from build123d import *

# Parameters (mm, degrees)
F0_W         = 70
F0_H         = 20
F0_R         = 5.25
F1_DEPTH     = 17.5
F2_T         = -3
F3_W         = 80
F3_H         = 53
F4_DEPTH     = 25
F5_T         = 2.5
F5_T3_DEPTH  = 40
F5_T5_DEPTH  = 75
F5_T7_DEPTH  = 69
F5_T9_DEPTH  = 22
F5_T11_DEPTH = 34


# Not quite as in the source:
# - a shell that OpenCascade refuses in one call is made with other operations: the cavity is built on its own and cut out


with BuildPart() as f1:
    # F0 (on Right) → F1 (new body, symmetric)
    with BuildSketch(Plane.YZ):
        Rectangle(F0_W, F0_H)
        with Locations((-22.5, 0)):
            Circle(F0_R, mode=Mode.SUBTRACT)
        with Locations((22.5, 0)):
            Circle(F0_R, mode=Mode.SUBTRACT)
    extrude(amount=F1_DEPTH, both=True)

    # F2
    f2_openings = [f1.faces().sort_by_distance(p)[0] for p in [
        (0, 0, 10),
        (0, -27.75, 0),
        (0, 17.25, 0),
    ]]
    offset(amount=F2_T, openings=f2_openings)

    # F3 (on Right) → F4 (join, symmetric)
    with BuildSketch(Plane.YZ):
        with Locations((0, 36.5)):
            Rectangle(F3_W, F3_H)
    extrude(amount=F4_DEPTH, both=True)

    # F5: shell of thickness 2.5, made by hand


with BuildPart() as f5_core1:
    # F5_t2: copy of F1
    add(f1.part)

    # the walls: a layer under each face that stays
    f5_faces = [f5_core1.faces().sort_by_distance(p)[0] for p in [
        (-21.4285714286, -34.2857142857, 10),
        (-25, 0, 36.5),
        (0, -40, 36.5),
        (0, 40, 36.5),
        (25, 0, 36.5),
        (0, 35, 0),
        (17.5, 0, 0),
        (0, -35, 0),
        (-17.5, 0, 0),
        (0, 0, -10),
        (16, -27.75, 0),
        (16, 17.25, 0),
        (-16, -27.75, 0),
        (-16, 17.25, 0),
        (14.5, 0, 1.5),
        (-14.5, 0, 1.5),
        (0, 0, 10),
        (0, -32, 1.5),
        (0, 0, -7),
        (0, 32, 1.5),
    ]]
    thicken(f5_faces, amount=-F5_T, mode=Mode.SUBTRACT)

    # F5_s4 → F5_t3 (cut)
    with BuildSketch(Plane.YZ.offset(-20)):
        Polygon((35.025, 9.975), (35, 12.5), (32.5, 12.5), (32.5, 10), align=None)
        Polygon((-35.025, 9.975), (-35, 12.5), (-32.5, 12.5), (-32.5, 10), align=None)
    extrude(amount=F5_T3_DEPTH, mode=Mode.SUBTRACT)

    # F5_s6 → F5_t5 (cut)
    with BuildSketch(Plane.XZ.offset(-37.5)):
        Polygon((17.525, 9.975), (17.5, 12.5), (15, 12.5), (15, 10), align=None)
        Polygon((-17.525, 9.975), (-17.5, 12.5), (-15, 12.5), (-15, 10), align=None)
    extrude(amount=F5_T5_DEPTH, mode=Mode.SUBTRACT)

    # F5_s8 → F5_t7 (cut)
    with BuildSketch(Plane.XZ.offset(-34.5)):
        Polygon((14.475, 9.975), (17, 10), (17, 12.5), (14.5, 12.5), align=None)
        Polygon((14.475, -6.975), (17, -7), (17, -9.5), (14.5, -9.5), align=None)
        Polygon((-14.475, 9.975), (-17, 10), (-17, 12.5), (-14.5, 12.5), align=None)
        Polygon((-14.475, -6.975), (-17, -7), (-17, -9.5), (-14.5, -9.5), align=None)
    extrude(amount=F5_T7_DEPTH, mode=Mode.SUBTRACT)

    # F5_s10 → F5_t9 (cut)
    with BuildSketch(Plane.XY.offset(-9.5)):
        Polygon((14.475, -31.975), (17, -32), (17, -34.5), (14.5, -34.5), align=None)
        Polygon((14.475, 31.975), (17, 32), (17, 34.5), (14.5, 34.5), align=None)
        Polygon((-14.475, -31.975), (-17, -32), (-17, -34.5), (-14.5, -34.5), align=None)
        Polygon((-14.475, 31.975), (-17, 32), (-17, 34.5), (-14.5, 34.5), align=None)
    extrude(amount=F5_T9_DEPTH, mode=Mode.SUBTRACT)

    # F5_s12 → F5_t11 (cut)
    with BuildSketch(Plane.YZ.offset(-17)):
        Polygon((-31.975, 9.975), (-32, 12.5), (-34.5, 12.5), (-34.5, 10), align=None)
        Polygon((31.975, 9.975), (32, 12.5), (34.5, 12.5), (34.5, 10), align=None)
        Polygon((-31.975, -6.975), (-34.5, -7), (-34.5, -9.5), (-32, -9.5), align=None)
        Polygon((31.975, -6.975), (32, -9.5), (34.5, -9.5), (34.5, -7), align=None)
    extrude(amount=F5_T11_DEPTH, mode=Mode.SUBTRACT)


with BuildPart() as f1_1:
    add(f1.part)

    # what is left inside the walls is the cavity
    f5_cavity = [f5_core1.part.solids().sort_by_distance(p)[0] for p in [
        (22.475, 0, 29.333333),
    ]]
    add(f5_cavity, mode=Mode.SUBTRACT)


solid = f1_1.part
Verification items for the finished model (mm, model axes). A direction names the side the tool comes from. Give positions to 0.01 mm unless a question says otherwise; leave off trailing zeros. Write each loop counter-clockwise with the first axis right and the second up, starting at its lowest first coordinate (ties: lowest second). Pieces come first, ordered by that corner, then holes. Notation, with made-up numbers: M 53.25,-15 L 57.25,-15 A29 ccw 57.25,8 Z; hole C 63,68.5 d8. An arc over 180 degrees is marked long. Write item = value, one per line.
(1) Sectioned sample at D-D (x = -9.5). Record the cut outline in (y, z).
Found:
outline = M -40,10 L -35,10 L -35,-10 L 35,-10 L 35,10 L 40,10 L 40,63 L 37.5,63 L 37.5,12.5 L -37.5,12.5 L -37.5,63 L -40,63 Z; hole M -32,-7 L 32,-7 L 32,10 L -32,10 Z
(2) Draft check along Y on faces 5 (the face through (0, 37.5, 37)), 6 (the face through (0, 40, 36)), 7 (the face through (-18, -3, 10)). Enter one of: released by +Y, released by -Y, zero draft, split by the parting line, or undercut.
Found:
face_5 = undercut
face_6 = released by +Y
face_7 = zero draft
(3) Sectioned sample at A-A (x = 15.5). Record the cut outline in (y, z).
Found:
outline = M -40,10 L -35,10 L -35,-10 L 35,-10 L 35,10 L 40,10 L 40,63 L 37.5,63 L 37.5,12.5 L -37.5,12.5 L -37.5,63 L -40,63 Z; hole C -22.5,0 d10.5; hole C 22.5,0 d10.5
(4) Material ranges on line 1 (Y direction, x = -20, z = 23.5); line 2 (Z direction, x = -15.9, y = -22.5); line 3 (Y direction, x = 12.5, z = -4.5), recorded low to high.
Found:
line_1 = -40 to -37.5, 37.5 to 40
line_2 = -10 to -5.25, 5.25 to 12.5
line_3 = -35 to -32, 32 to 35
(5) Sectioned sample at B-B (z = 0). Record the cut outline in (x, y).
Found:
outline = M -17.5,-35 L 17.5,-35 L 17.5,-27.75 L 14.5,-27.75 L 14.5,-32 L -14.5,-32 L -14.5,-27.75 L -17.5,-27.75 Z; M -17.5,-17.25 L -14.5,-17.25 L -14.5,17.25 L -17.5,17.25 Z; M -17.5,27.75 L -14.5,27.75 L -14.5,32 L 14.5,32 L 14.5,27.75 L 17.5,27.75 L 17.5,35 L -17.5,35 Z; M 14.5,-17.25 L 17.5,-17.25 L 17.5,17.25 L 14.5,17.25 Z
(6) Sectioned sample at C-C (y = -22.5). Record the cut outline in (x, z).
Found:
outline = M -25,10 L -17.5,10 L -17.5,5.25 L -14.5,5.25 L -14.5,10 L 14.5,10 L 14.5,5.25 L 17.5,5.25 L 17.5,10 L 25,10 L 25,63 L 22.5,63 L 22.5,12.5 L -22.5,12.5 L -22.5,63 L -25,63 Z; M -17.5,-10 L 17.5,-10 L 17.5,-5.25 L 14.5,-5.25 L 14.5,-7 L -14.5,-7 L -14.5,-5.25 L -17.5,-5.25 Z
(7) Go/stop test with flat-tipped pins: pin 1 Ø6 at (y, z) = (-8, 1) entering from -X; pin 2 Ø13.5 at (y, z) = (2.5, -2) entering from +X; pin 3 Ø6 at (x, y) = (6, -30) entering from +Z. Record where each tip stops, or that it passes through.
Found:
pin_1 = -17.5
pin_2 = 17.5
pin_3 = 12.5
(8) Access from +Z, -Z, +X, -X, +Y, -Y to the whole of each face (thin tool, end or side, straight path). Record for faces 1 (the face through (14.5, 0, 2)), 2 (the face through (0, 35, 0)), 3 (the face through (22.5, -1, 38)), 4 (the face through (0, -35, 0)).
Found:
face_1 = none
face_2 = -Z, +X, -X, +Y
face_3 = +Z
face_4 = -Z, +X, -X, -Y
